CAD build for the part. Positions are in the model's coordinates, mm. Face numbers are marked on the shaded views. A direction names the side the tool comes from. Round coordinates to 2 decimals unless told otherwise and drop trailing zeros. Write each loop counter-clockwise with the first axis right and the second up, starting at its lowest first coordinate (ties: lowest second). Pieces come first, ordered by that corner, then holes. Notation, with made-up numbers: (-5.5, 64.25) - (36.5, 64.25) arc R17 ccw to (36.5, 97.25) - close; hole circle Ø10 at (19, 50). An arc over 180 degrees is marked (long way). Answer in a Markdown table with one row per item.
```python
from build123d import *

# Parameters (mm, degrees)
SKETCH_1_R               = 56.885850613
SKETCH_1_R_2             = 31.885850613
EXTRUDE_1_DEPTH          = 25
FILLET_1_R               = 5
SKETCH_2_W               = 13
SKETCH_2_H               = 10
SKETCH_2_R               = 2.25
EXTRUDE_1_2_DEPTH        = 15
PATTERN_CIRCULAR_1_COUNT = 4


with BuildPart() as part:
    # Эскиз1 → Extrude 1 (new body)
    with BuildSketch(Plane(origin=(0, 0, 16.5), x_dir=(1, 0, 0), z_dir=(0, 1, 0))):
        with Locations((0, 16.5)):
            Circle(SKETCH_1_R)
        with Locations((0, 16.5)):
            Circle(SKETCH_1_R_2, mode=Mode.SUBTRACT)
    extrude(amount=EXTRUDE_1_DEPTH)

    # Скругление1
    fillet_1_edges = [part.edges().sort_by_distance(p)[0] for p in [
        (-56.885850613, 0, 0),
        (-56.885850613, 25, 0),
        (-31.885850613, 0, 0),
        (-31.885850613, 25, 0),
    ]]
    fillet(fillet_1_edges, radius=FILLET_1_R)

    # Эскиз2 → Extrude 1 2 (add)
    with BuildSketch(Plane.XZ):
        with Locations((-41.9, 0)):
            Rectangle(SKETCH_2_W, SKETCH_2_H)
        with Locations(Location((-41.9, 0, 0), (0, 0, 270))):
            Circle(SKETCH_2_R, mode=Mode.SUBTRACT)
    extrude_1_2 = extrude(amount=EXTRUDE_1_2_DEPTH)

    # Круговой массив1: Extrude 1 2 ×4 about axis
    pattern_circular_1_axis = Axis((0, 0, 0), (0, 1, 0))
    for i in range(1, PATTERN_CIRCULAR_1_COUNT):
        add(extrude_1_2.rotate(pattern_circular_1_axis, i * 360 / PATTERN_CIRCULAR_1_COUNT))


solid = part.part
```
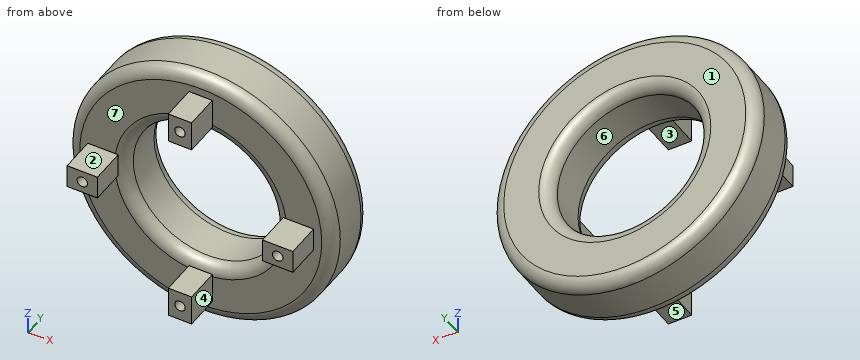
Q1. Pull direction Z, two halves, no side cores. Call the marked faces 5, 6 and 7: released by +Z, released by -Z, zero draft, split by the parting line, or undercut.
Computed:
| item | result |
|---|---|
| face 5 | released by -Z |
| face 6 | undercut |
| face 7 | zero draft |
Q2. Flat gauge pins, fed straight in: pin 1 (6.5 mm diameter, centred on y = -4, z = -44, fed in from -X); pin 2 (12 mm diameter, centred on x = 43.5, z = 20, fed in from -Y); pin 3 (5 mm diameter, centred on x = 2, y = -6, fed in from -Z); pin 4 (5 mm diameter, centred on x = 41, z = -0.5, fed in from -Y). Where does each tip first touch, or does it go through?
Computed:
| item | result |
|---|---|
| pin 1 | stops at x = -5 |
| pin 2 | stops at y = 0 |
| pin 3 | stops at z = -48.4 |
| pin 4 | stops at y = -15 |
Q3. Saw through at D-D on y = 7. List the corners of the cut face in (x, z), then the cut area to 3 significant figures.
Computed:
| item | result |
|---|---|
| outline | circle Ø113.77 at (0, 0); hole circle Ø63.77 at (0, 0) |
| area | 6,970 mm2 |
Q4. Saw through at A-A on y = -8. List the corners of the cut face in (x, z).
Computed:
| item | result |
|---|---|
| outline | (-48.4, -5) - (-35.4, -5) - (-35.4, 5) - (-48.4, 5) - close; (-5, -48.4) - (5, -48.4) - (5, -35.4) - (-5, -35.4) - close; (-5, 35.4) - (5, 35.4) - (5, 48.4) - (-5, 48.4) - close; (35.4, -5) - (48.4, -5) - (48.4, 5) - (35.4, 5) - close; hole circle Ø4.5 at (-41.9, 0); hole circle Ø4.5 at (0, -41.9); hole circle Ø4.5 at (0, 41.9); hole circle Ø4.5 at (41.9, 0) |
Q5. Drill centre lines: line 1 (X direction, y = -6.5, z = 0); line 2 (Z direction, x = 0, y = 13). Where is each one in solid material? Low to high.
Computed:
| item | result |
|---|---|
| line 1 | x = -48.4 to -44.15, -39.65 to -35.4, 35.4 to 39.65, 44.15 to 48.4 |
| line 2 | z = -56.89 to -31.89, 31.89 to 56.89 |
Q6. 3-axis set-ups, long thin cutter, end or side, ignore diameter. For the marked faces 1, 2, 3 and 4: which of +Z, -Z, +X, -X, +Y, -Y reach the whole face in a straight line?
Computed:
| item | result |
|---|---|
| face 1 | +Z, -Z, +X, -X, +Y |
| face 2 | +Z, +X, -X, -Y |
| face 3 | +X, -X, -Y |
| face 4 | +Z, -Z, +X, -Y |
